The listing builds one solid part. Answer for the finished solid, in the listing's coordinates (mm). Face numbers are marked on the shaded views. Give positions to 0.01 mm unless a question says otherwise; leave off trailing zeros. Loops run counter-clockwise (first coordinate to the right, second up) from the corner with the lowest first, then second, coordinate; pieces in that order, holes last. Notation, with made-up numbers: (88, -35.75) - (114, -35.75) arc R22 cw to (114, -18.75) - close; hole circle Ø9 at (31.25, 37). An arc over 180 degrees is marked (long way). Answer as CSV lines item,"result". Start each with the question number.
1) A cutting plane is placed at B-B (y = 0). Determine the outline of the cut face in (x, z), and give its area (3 significant figures).
2) Flat-ended cylindrical pins translate along their axes: pin 1 (2 mm diameter, centred on x = -1, z = -19, fed in from -Y); pin 2 (4 mm diameter, centred on y = -4, z = -11.5, fed in from +X); pin 3 (2 mm diameter, centred on x = -3, z = -3.5, fed in from -Y); pin 4 (1.6 mm diameter, centred on x = 0, y = 0, fed in from -Z). Find the tip coordinate at first contact, or state that the pin passes through.
3) Find the intervals of material crossed by line 1 along X through (y, z) = (0, -22.5); line 2 along Z through (x, y) = (-4.5, 3.75); line 3 along X through (y, z) = (-1, -21), in increasing order.
4) For a pull along Y with two mould halves and no side action, classify the marked faces 1, 2 and 3 as pulls with the +Y half, pulls with the -Y half, needs draft (parallel to the pull), parting line crosses it, or undercut.
5) A cutting plane is placed at C-C (z = -10). Determine the outline of the cut face in (x, y), and give its area (3 significant figures).
```python
from build123d import *

# Parameters (mm, degrees)
CUT_EXTRUDE1_DEPTH = 26.2


with BuildPart() as part:
    # Sketch1 → Revolve1 (revolve)
    with BuildSketch(Plane(origin=(0, 0, 0), x_dir=(0, 0, -1), z_dir=(1, 0, 0))):
        with BuildLine():
            Line((0, 5.078211692), (0, 6.1))
            Line((0, 6.1), (1, 6.1))
            Line((1, 6.1), (1, 5.8))
            ThreePointArc((1, 5.8), (2.025126266, 3.325126266), (4.5, 2.3))
            Line((4.5, 2.3), (9.440083729, 2.3))
            Line((9.440083729, 2.3), (9.440083729, 2.8))
            Line((9.440083729, 2.8), (10.940083729, 2.8))
            Line((10.940083729, 2.8), (10.940083729, 2.3))
            Line((10.940083729, 2.3), (26.140083729, 2.3))
            Line((26.140083729, 2.3), (26.140083729, 2.8))
            Line((26.140083729, 2.8), (27.640083729, 2.8))
            Line((27.640083729, 2.8), (27.640083729, 2.3))
            Line((27.640083729, 2.3), (28.853856016, 2.3))
            Line((28.853856016, 2.3), (28.853856016, 1.3))
            Line((28.853856016, 1.3), (4.548739728, 1.3))
            ThreePointArc((4.548739728, 1.3), (2.968613199, 1.676988608), (1.728880785, 2.72674277))
            Line((1.728880785, 2.72674277), (0, 5.078211692))
        make_face()
    revolve(axis=Axis((0, 0, 0), (0, 0, -1)))

    # Sketch2 → Cut-Extrude1 (cut)
    with BuildSketch(Plane.XY):
        Polygon((2, 6), (2, -6.569031419), (7.819181693, -6.569031419), (7.708002274, 5.9580813), align=None)
    extrude(amount=-CUT_EXTRUDE1_DEPTH, mode=Mode.SUBTRACT)


solid = part.part
```
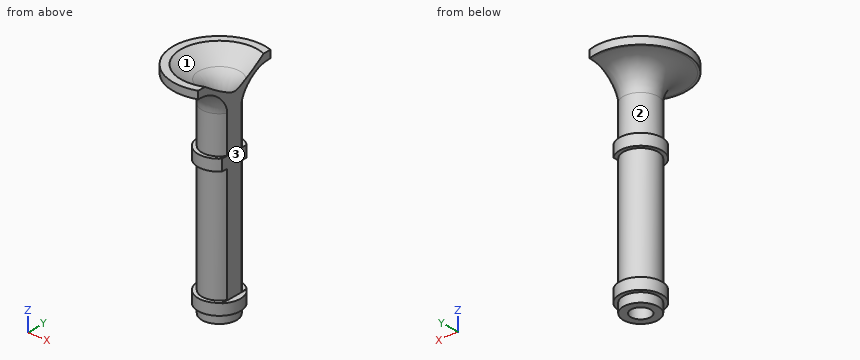
Ans:
1,outline,"(-6.1, -1) - (-5.8, -1) arc R3.5 cw to (-2.3, -4.5) - (-2.3, -9.44) - (-2.8, -9.44) - (-2.8, -10.94) - (-2.3, -10.94) - (-2.3, -26.14) - (-2.8, -26.14) - (-2.8, -27.64) - (-2.3, -27.64) - (-2.3, -28.85) - (-1.3, -28.85) - (-1.3, -4.55) arc R3.5 ccw to (-2.73, -1.73) - (-5.08, 0) - (-6.1, 0) - close; (1.3, -28.85) - (2.3, -28.85) - (2.3, -27.64) - (2.8, -27.64) - (2.8, -26.2) - (2, -26.2) - (2, -2.45) arc R3.5 ccw to (1.3, -4.55) - close"
1,area,"50.6 mm2"
2,pin 1,"y = -2.3"
2,pin 2,"x = 1.87"
2,pin 3,"y = -1.55"
2,pin 4,"through"
3,line 1,"-2.3 to -1.3, 1.3 to 2"
3,line 2,"-1 to 0"
3,line 3,"-2.07 to -0.83, 0.83 to 2"
4,face 1,"undercut"
4,face 2,"parting line crosses it"
4,face 3,"needs draft"
5,outline,"(2, -1.96) - (2, 1.96) arc R2.8 ccw (long way) to start; hole circle Ø2.6 at (0, 0)"
5,area,"17.2 mm2"
